Autodesk Inventor part; units mm, degrees
ref_plane "YZ Plane" through (0, 0, 0) normal (1, 0, 0) x (0, 1, 0)
ref_plane "XZ Plane" through (0, 0, 0) normal (0, 1, 0) x (-1, 0, 0)
ref_plane "XY Plane" through (0, 0, 0) normal (0, 0, 1) x (1, 0, 0)
sketch "スケッチ1" plane through (0, 0, 0) normal (0, 0, 1) x (1, 0, 0)
  circle A0 centre (0, 0) radius 4
  dimension "d0" = 8
extrude "押し出し1" add sketch "スケッチ1" along normal blind 159
sketch "スケッチ2" plane through (0, 0, 0) normal (0, 0, -1) x (-1, 0, 0)
  circle A0 centre (0, 0) radius 4
  circle A1 centre (0, 0) radius 1.25
  dimension "d3" = 2.5
extrude "押し出し2" cut sketch "スケッチ2" against normal blind 6 contours A1
sketch "スケッチ3" plane through (0, 0, 159) normal (0, 0, 1) x (1, 0, 0)
  circle A0 centre (0, 0) radius 4
  circle A1 centre (0, 0) radius 1.25
  circle A2 centre (0, 0) radius 1.25
  dimension "d6" = 2.5
extrude "押し出し3" cut sketch "スケッチ3" against normal blind 6 contours A1
properties part number "シャフト　ポリカ" material "ポリカーボネート、クリア"
Geometry: final body of the model. Coordinates: model frame, mm. A direction names the side the tool comes from. Coordinates: 2 decimals unless noted, no trailing zeros. Write each loop counter-clockwise with the first axis right and the second up, starting at its lowest first coordinate (ties: lowest second). Pieces come first, ordered by that corner, then holes. Notation, with made-up numbers: (-38.5, 54) - (3.5, 54) arc R30 ccw to (3.5, 87) - close; hole circle Ø9 at (74.25, 18). An arc over 180 degrees is marked (long way). Return JSON: item names as keys, results as strings.
Item 1: Pin query (flat end, axial travel): pin 1 Ø2 at (x, y) = (0, 0) entering from -Z; pin 2 Ø3 at (y, z) = (-3, 133.5) entering from -X. Return the tip coordinate at first contact, or that it passes through.
Completed:
{"pin 1": "stops at z = 6", "pin 2": "stops at x = -3.71"}
Item 2: Section query C-C (z = 76). Output: boundary loops of the cut face in (x, y).
Completed:
{"outline": "circle Ø8 at (0, 0)"}
Item 3: Pull-direction query (Y, two-part tool) for faces 4 (the face through (-1, -1, 159)), 5 (the face through (-0.867, 3.905, 78.387)), 6 (the face through (0.27, -1.22, 2.96)); classes: +Y half, -Y half, draft (parallel to the pull), parting line (faces both ways), or undercut.
Completed:
{"face 4": "draft", "face 5": "parting line", "face 6": "undercut"}
Item 4: Reachability of faces 1 (the face through (0, 0, 6)), 2 (the face through (-0.27, -1.22, 156.04)), 3 (the face through (-1, -1, 0)) from +Z, -Z, +X, -X, +Y, -Y: full face, straight path, thin tool, end or side. Return the list, or none.
Completed:
{"face 1": "-Z", "face 2": "+Z", "face 3": "-Z, +X, -X, +Y, -Y"}
Item 5: Section query A-A (y = 0). Output: boundary loops of the cut face in (x, z).
Completed:
{"outline": "(-4, 0) - (-1.25, 0) - (-1.25, 6) - (1.25, 6) - (1.25, 0) - (4, 0) - (4, 159) - (1.25, 159) - (1.25, 153) - (-1.25, 153) - (-1.25, 159) - (-4, 159) - close"}
Item 6: Line query: L1, parallel to Y at x = 0, z = 3.6; L2, parallel to X at y = 0.25, z = 140.5; L3, parallel to Z at x = -0.5, y = -0.5. Output: solid intervals per line, ascending.
Completed:
{"L1": "y = -4 to -1.25, 1.25 to 4", "L2": "x = -3.99 to 3.99", "L3": "z = 6 to 153"}
